Geometry check sheet. Reference: drawing and pictorial views, mm from the part's lowest x, y, z. Round coordinates to 2 decimals unless told otherwise and drop trailing zeros. Write each loop counter-clockwise with the first axis right and the second up, starting at its lowest first coordinate (ties: lowest second). Pieces come first, ordered by that corner, then holes. Notation, with made-up numbers: M 9.5,7.5 L 13.5,7.5 A20 ccw 13.5,23.5 Z; hole C 69,-28 d9. An arc over 180 degrees is marked long. Answer in a Markdown table with one row per item.
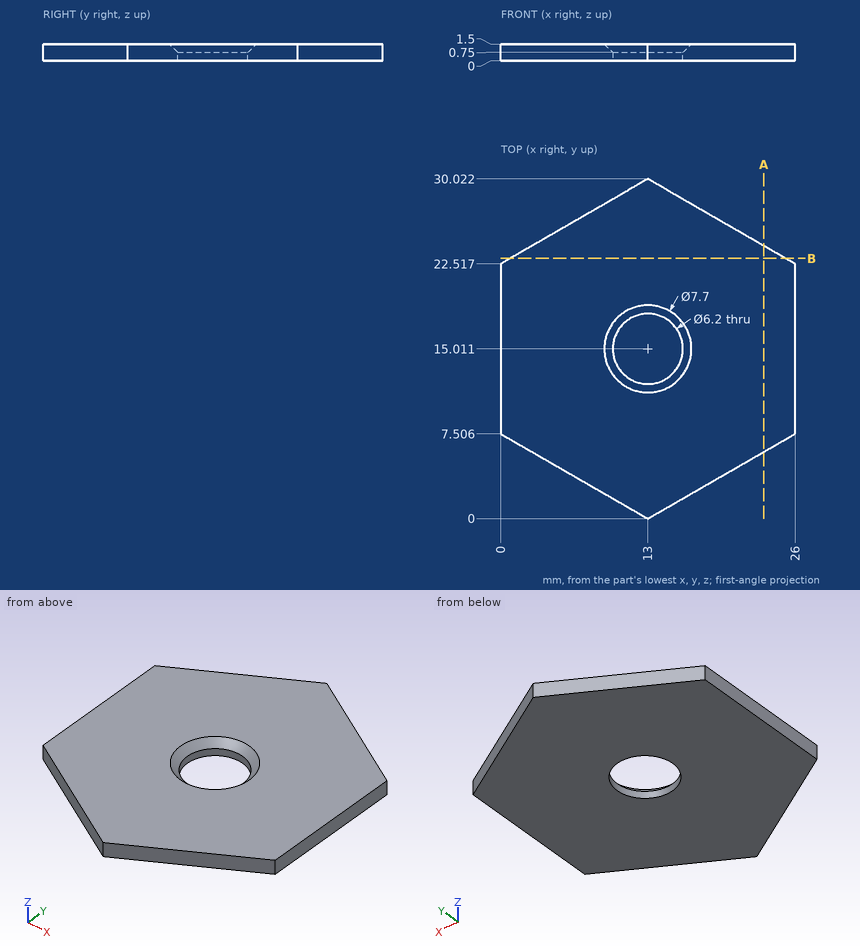
1. Go/stop test with flat-tipped pins: pin 1 (5 mm diameter, centred on x = 13, y = 15.01, fed in from -Z); pin 2 (2 mm diameter, centred on x = 18, y = 11.5, fed in from -Z). Record where each tip stops, or that it passes through.
Found:
| item | result |
|---|---|
| pin 1 | passes through |
| pin 2 | stops at z = 0 |
2. Section check B-B, the plane y = 23. Record the cut outline in (x, z).
Found:
| item | result |
|---|---|
| outline | M 0.84,0 L 25.16,0 L 25.16,1.5 L 0.84,1.5 Z |
3. Section check A-A, the plane x = 23.25. Record the cut outline in (y, z) (1 decimal).
Found:
| item | result |
|---|---|
| outline | M 5.9,0 L 24.1,0 L 24.1,1.5 L 5.9,1.5 Z |
4. Scan lines: L1, parallel to Y at x = 15.25, z = 1.4 (1 decimal); L2, parallel to Y at x = 13.5, z = 1.25 (1 decimal); L3, parallel to X at y = 14, z = 0.15. Record each from-to range of solid material in increasing order.
Found:
| item | result |
|---|---|
| L1 | y = 1.3 to 12, 18 to 28.7 |
| L2 | y = 0.3 to 11.4, 18.6 to 29.7 |
| L3 | x = 0 to 10.07, 15.93 to 26 |
